from build123d import *

# Parameters (mm, degrees)
CROQUIS1_W              = 316
CROQUIS1_H              = 433
SALIENTE_EXTRUIR3_DEPTH = 1
CROQUIS2_W              = 314
CROQUIS2_H              = 431
SALIENTE_EXTRUIR4_DEPTH = 20
CROQUIS3_R              = 2
SALIENTE_EXTRUIR5_DEPTH = 10
CROQUIS4_R              = 2.5
CORTAR_EXTRUIR1_DEPTH   = 316
CROQUIS5_R              = 3
CORTAR_EXTRUIR2_DEPTH   = 1


with BuildPart() as part:
    # Croquis1 → Saliente-Extruir3 (new body)
    with BuildSketch(Plane.XY):
        with Locations((-158, 216.5)):
            Rectangle(CROQUIS1_W, CROQUIS1_H)
    extrude(amount=SALIENTE_EXTRUIR3_DEPTH)

    # Croquis2 → Saliente-Extruir4 (add)
    with BuildSketch(Plane.XY.offset(1)):
        Polygon((-315, 433), (-316, 433), (-316, 432), (-316, 1), (-316, 0), (-315, 0), (-1, 0), (0, 0), (0, 1), (0, 432), (0, 433), align=None)
        with Locations((-158, 216.5)):
            Rectangle(CROQUIS2_W, CROQUIS2_H, mode=Mode.SUBTRACT)
    extrude(amount=SALIENTE_EXTRUIR4_DEPTH)

    # Croquis3 → Saliente-Extruir5 (add)
    with BuildSketch(Plane.XY.offset(1)):
        with Locations((-287, 376)):
            Circle(CROQUIS3_R)
        with Locations((-29, 376)):
            Circle(CROQUIS3_R)
        with Locations((-287, 79)):
            Circle(CROQUIS3_R)
        with Locations((-29, 79)):
            Circle(CROQUIS3_R)
    extrude(amount=SALIENTE_EXTRUIR5_DEPTH)

    # Croquis4 → Cortar-Extruir1 (cut)
    with BuildSketch(Plane(origin=(0, 0, 0), x_dir=(0, 0, -1), z_dir=(1, 0, 0))):
        with Locations((-10, 366.5)):
            Circle(CROQUIS4_R)
        with Locations((-10, 66.5)):
            Circle(CROQUIS4_R)
        with Locations((-10, 216.5)):
            Circle(CROQUIS4_R)
    extrude(amount=-CORTAR_EXTRUIR1_DEPTH, mode=Mode.SUBTRACT)

    # Croquis5 → Cortar-Extruir2 (cut)
    with BuildSketch(Plane.XY.offset(1)):
        with Locations((-298, 412.5)):
            Circle(CROQUIS5_R)
        with Locations((-298, 20.5)):
            Circle(CROQUIS5_R)
        with Locations((-18, 412.5)):
            Circle(CROQUIS5_R)
        with Locations((-18, 20.5)):
            Circle(CROQUIS5_R)
    extrude(amount=-CORTAR_EXTRUIR2_DEPTH, mode=Mode.SUBTRACT)


solid = part.part
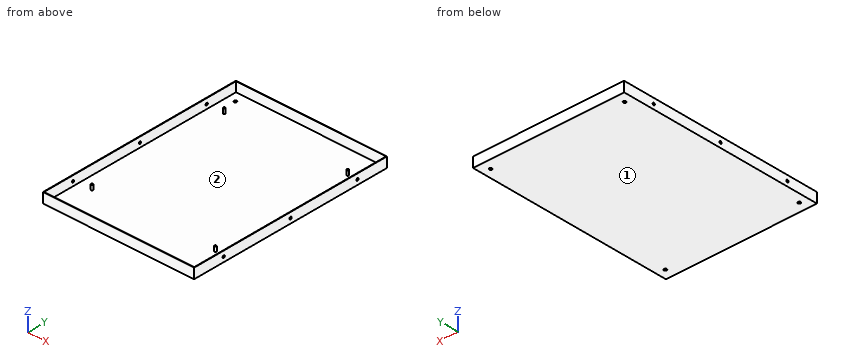
Verification items for the finished model (mm, model axes). Face numbers are marked on the shaded views. Round coordinates to 2 decimals unless told otherwise and drop trailing zeros. Order: outer loops, then holes, each group sorted by start corner. A loop starts at its lowest first (then second) coordinate and runs counter-clockwise, first axis right, second up.
1. Section check C-C on y = 188. Record the cut outline in (x, z).
Final values:
outline: (-316, 0) - (0, 0) - (0, 21) - (-1, 21) - (-1, 1) - (-315, 1) - (-315, 21) - (-316, 21) - close
2. Section check B-B on x = -213.5. Record the cut outline in (y, z), then the cut area to 3 significant figures.
Final values:
outline: (0, 0) - (433, 0) - (433, 21) - (432, 21) - (432, 1) - (1, 1) - (1, 21) - (0, 21) - close
area: 473 mm2
3. Go/stop test with flat-tipped pins: P1, Ø4.5, axis at x = -286, y = 377, coming from the +Z side; P2, Ø3, axis at y = 216.5, z = 10, coming from the -X side; P3, Ø5, axis at x = -275.5, y = 263.5, coming from the +Z side. Record where each tip stops, or that it passes through.
Final values:
P1: stops at z = 11
P2: passes through
P3: stops at z = 1
4. Section check A-A on z = 15.75. Record the cut outline in (x, y), then the cut area to 3 significant figures.
Final values:
outline: (-316, 0) - (0, 0) - (0, 433) - (-316, 433) - close; hole (-315, 1) - (-1, 1) - (-1, 432) - (-315, 432) - close
area: 1,490 mm2
5. Thickness scan on L1, parallel to Y at x = -18, z = 0.6; L2, parallel to Y at x = -315.65, z = 10; L3, parallel to Y at x = -40, z = 4. Record the ranges inside material, lowest first.
Final values:
L1: y = 0 to 17.5, 23.5 to 409.5, 415.5 to 433
L2: y = 0 to 64, 69 to 214, 219 to 364, 369 to 433
L3: y = 0 to 1, 432 to 433
6. Release check for a two-part mould opening along Y. For the marked faces 1 and 2 record: +Y half, -Y half, draft (parallel to the pull), parting line (faces both ways), or undercut.
Final values:
face 1: draft
face 2: undercut
